from build123d import *

# Parameters (mm, degrees)
SKETCH1_W             = 30.1
SKETCH1_H             = 1.52
BOSS_EXTRUDE1_DEPTH   = 16.1
BOSS_EXTRUDE2_START   = 3.6
SKETCH2_W             = 12.88
SKETCH2_H             = 7.56
BOSS_EXTRUDE2_DEPTH   = 3.68
BOSS_EXTRUDE2_DRAFT   = 10
BOSS_EXTRUDE3_START   = -11.337254685
BOSS_EXTRUDE3_DEPTH   = 5.63450937
BOSS_EXTRUDE3_START_2 = 17.89
BOSS_EXTRUDE3_2_DEPTH = 7.204859471
BOSS_EXTRUDE3_START_3 = 1
BOSS_EXTRUDE3_3_DEPTH = 5.72461499
FILLET1_R             = 3


with BuildPart() as part:
    # Sketch1 → Boss-Extrude1 (new body)
    with BuildSketch(Plane.XY):
        with Locations((15.05, 0.76)):
            Rectangle(SKETCH1_W, SKETCH1_H)
    extrude(amount=-BOSS_EXTRUDE1_DEPTH)


with BuildPart() as boss_extrude2_tool:
    # Sketch2 → Boss-Extrude2 (with draft: the straight prism first)
    with BuildSketch(Plane(origin=(0, 1.52, 0), x_dir=(1, 0, 0), z_dir=(0, 1, 0)).offset(BOSS_EXTRUDE2_START)):
        with Locations((11.45, 8.52)):
            Rectangle(SKETCH2_W, SKETCH2_H)
    extrude(amount=-BOSS_EXTRUDE2_DEPTH)
    # Boss-Extrude2: the draft: its side faces are tilted about the plane it starts from
    boss_extrude2_sides = [boss_extrude2_tool.faces().sort_by_distance(p)[0] for p in [
        (5.01, 3.28, -8.52),
        (11.45, 3.28, -4.74),
        (17.89, 3.28, -8.52),
        (11.45, 3.28, -12.3),
    ]]
    draft(boss_extrude2_sides, Plane(origin=(0, 1.52, 0), x_dir=(1, 0, 0), z_dir=(0, 1, 0)).offset(BOSS_EXTRUDE2_START), BOSS_EXTRUDE2_DRAFT)


with BuildPart() as part_1:
    add(part.part)

    # Boss-Extrude2: add boss_extrude2_tool
    add(boss_extrude2_tool.part)

    # Boss-Extrude3: read off the stored shape, not the designer's step
    # Boss-Extrude3 outline → Boss-Extrude3 (add)
    with BuildSketch(Plane.XY.offset(BOSS_EXTRUDE3_START)):
        Polygon((18.524777131, 1.52), (25.094859471, 1.52), (25.094859471, 10.58), (17.89, 5.12), align=None)
    extrude(amount=BOSS_EXTRUDE3_DEPTH)

    # Boss-Extrude3 2 outline → Boss-Extrude3 2 (add)
    with BuildSketch(Plane.YZ.offset(BOSS_EXTRUDE3_START_2)):
        Polygon((1.52, -11.337254685), (1.52, -12.934777131), (10.58, -11.337254685), align=None)
        Polygon((1.52, -4.105222869), (1.52, -5.702745315), (10.58, -5.702745315), align=None)
    extrude(amount=BOSS_EXTRUDE3_2_DEPTH)

    # Boss-Extrude3 3 outline → Boss-Extrude3 3 (cut)
    with BuildSketch(Plane(origin=(0, 0, 0), x_dir=(0.7969977291170371, 0.6039823008849562, 0), z_dir=(0.6039823008849562, -0.7969977291170373, 0)).offset(BOSS_EXTRUDE3_START_3)):
        Polygon((26.390678754, -11.337254685), (26.390678754, -5.702745315), (17.350678754, -4.74), (17.350678754, -12.3), align=None)
    extrude(amount=BOSS_EXTRUDE3_3_DEPTH, mode=Mode.SUBTRACT)

    # Fillet1
    fillet1_edges = [part_1.edges().sort_by_distance(p)[0] for p in [
        (11.45, 1.52, -4.105222869),
        (11.45, 1.52, -12.934777131),
        (4.375222869, 1.52, -8.52),
        (25.094859471, 1.52, -8.52),
    ]]
    fillet(fillet1_edges, radius=FILLET1_R)


solid = part_1.part
Read the model definition and answer for the solid it produces. Units are mm, in the model's axes. A direction names the side the tool comes from. Round coordinates to 2 decimals unless told otherwise and drop trailing zeros. Write each loop counter-clockwise with the first axis right and the second up, starting at its lowest first coordinate (ties: lowest second). Pieces come first, ordered by that corner, then holes.
Q1. Find section A-A on x = 10.5. Determine the outline of the cut face in (y, z), and give its area (3 significant figures).
Values:
outline: (0, -16.1) - (1.52, -16.1) - (1.52, -15.45) arc R3 cw to (4, -12.5) - (5.12, -12.3) - (5.12, -4.74) - (4, -4.54) arc R3 cw to (1.52, -1.59) - (1.52, 0) - (0, 0) - close
area: 56.5 mm2
Q2. Straight lines are drawn through the part: line 1 (Y direction, x = 16, z = -7.25); line 2 (Y direction, x = 7.5, z = -0.75); line 3 (Z direction, x = 21, y = 4). For each, find the intervals that lie inside material, in ascending order.
Values:
line 1: y = 0 to 5.12
line 2: y = 0 to 1.52
line 3: z = -12.5 to -4.54
Q3. Find section D-D on z = -15. Determine the outline of the cut face in (x, y), and give its area (3 significant figures).
Values:
outline: (0, 0) - (30.1, 0) - (30.1, 1.52) - (28.09, 1.52) arc R3 cw to (27.64, 1.55) - (2.31, 1.55) arc R3 cw to (1.86, 1.52) - (0, 1.52) - close
area: 46.6 mm2
Q4. Find section C-C on y = 8.25. Determine the outline of the cut face in (x, z).
Values:
outline: (22.02, -11.75) - (25.09, -11.75) - (25.09, -5.29) - (22.02, -5.29) - close
Q5. Find section B-B on z = -8.5. Determine the outline of the cut face in (x, y).
Values:
outline: (0, 0) - (30.1, 0) - (30.1, 1.52) - (28.09, 1.52) arc R3 cw to (25.09, 4.52) - (25.09, 10.58) - (17.89, 5.12) - (5.01, 5.12) - (4.81, 4) arc R3 cw to (1.86, 1.52) - (0, 1.52) - close
Q6. Flat-ended cylindrical pins translate along their axes: P1, Ø6, axis at x = 13, z = -9.5, coming from the +Y side; P2, Ø4, axis at y = 7, z = -3.5, coming from the +X side; P3, Ø2, axis at x = 9.5, y = 3, coming from the -Z side; P4, Ø4, axis at y = 8, z = -3, coming from the +X side. Find the tip coordinate at first contact, or state that the pin passes through.
Values:
P1: stops at y = 5.12
P2: stops at x = 25.09
P3: stops at z = -13.82
P4: passes through
Q7. A tool of negligible diameter and unlimited length cuts with its end or side. For faces 1 (the face through (11, 5.12, -9)), 2 (the face through (13, 1.52, -1)), 3 (the face through (25.095, 8, -8)), 4 (the face through (15, 1, 0)), from which of +Z, -Z, +X, -X, +Y, -Y can it reach the whole face along a straight path? Write none if from no direction.
Values:
face 1: +Z, -Z, -X, +Y
face 2: +Y
face 3: +Z, -Z, +X, +Y
face 4: +Z, +X, -X, +Y, -Y
